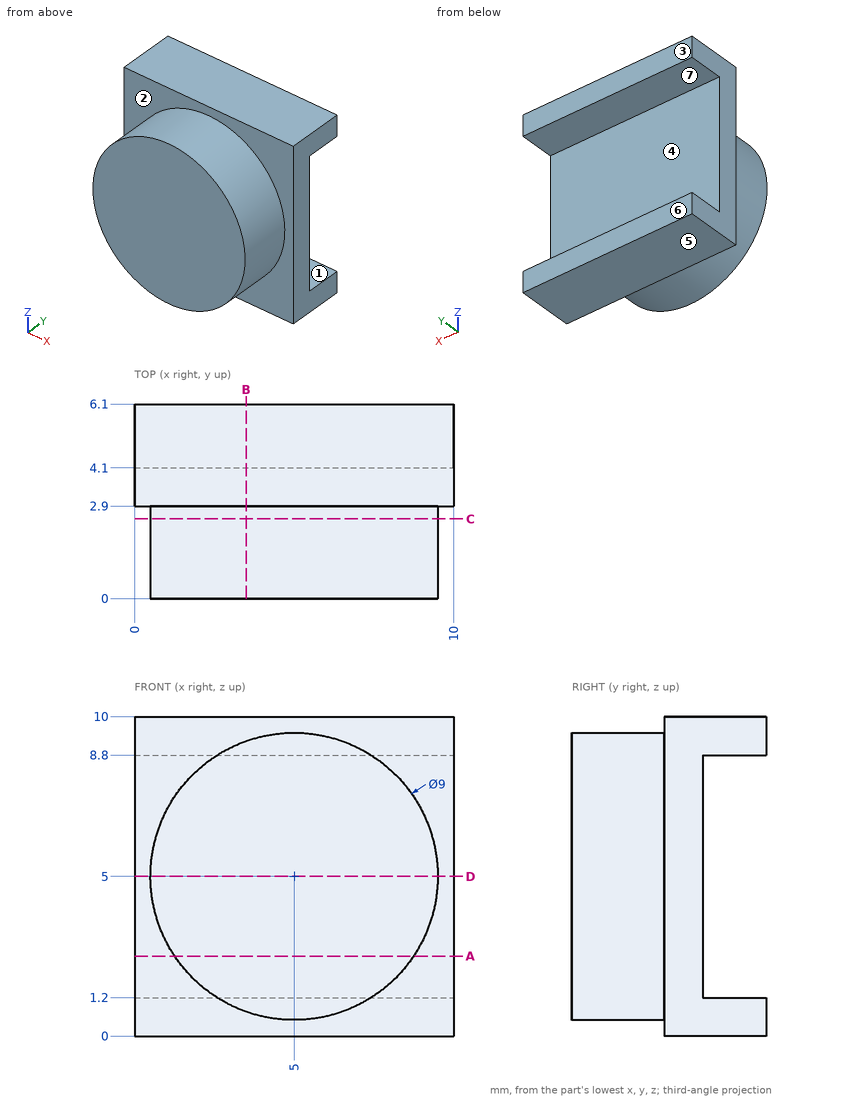
For this review, use the dimensioned drawing (mm, ordinates from the lowest corner) and the shaded views. A direction names the side the tool comes from. Give positions to 0.01 mm unless a question says otherwise; leave off trailing zeros. Loops run counter-clockwise (first coordinate to the right, second up) from the corner with the lowest first, then second, coordinate; pieces in that order, holes last.
Item 1: Take a section at D-D, the plane z = 5. State the section outline as (x, y) points.
Item 2: Tool access review of the marked faces 1, 2 and 3: name each direction out of +Z, -Z, +X, -X, +Y, -Y from which nothing blocks a thin tool from reaching the whole face with its end or side.
Item 3: Take a section at B-B, the plane x = 3.5. State the section outline as (y, z) points, and give its area (3 significant figures).
Item 4: Draft analysis for pull direction Z (two halves, no side actions). For the marked faces 4, 5, 6 and 7, state which applies: +Z half, -Z half, draft (parallel to the pull), parting line (faces both ways), or undercut.
Item 5: Take a section at A-A, the plane z = 2.5. State the section outline as (x, y) points, and give its area (3 significant figures).
Item 6: For line 1 along Z through (x, y) = (6.75, 5.5); line 2 along X through (y, z) = (1, 5); line 3 along Y through (x, z) = (4.5, 2.5), list the stretches that pass through material, from the lowest coordinate up.
Item 7: Take a section at C-C, the plane y = 2.5. State the section outline as (x, z) points.
Item 8: Insertion check: pin 1 (3 mm diameter, centred on x = 6.5, z = 5.5, fed in from +Y). The pin has a flat end and moves straight along its axis. Give the tip position at first contact, or say it passes through.
Calculated:
1. outline: (0, 2.9) - (0.5, 2.9) - (0.5, 0) - (9.5, 0) - (9.5, 2.9) - (10, 2.9) - (10, 4.1) - (0, 4.1) - close
2. face 1: +X, -X, +Y
2. face 2: -Y
2. face 3: +Z, -Z, +X, -X, +Y
3. outline: (0, 0.76) - (2.9, 0.76) - (2.9, 0) - (6.1, 0) - (6.1, 1.2) - (4.1, 1.2) - (4.1, 8.8) - (6.1, 8.8) - (6.1, 10) - (2.9, 10) - (2.9, 9.24) - (0, 9.24) - close
3. area: 41.4 mm2
4. face 4: undercut
4. face 5: -Z half
4. face 6: draft
4. face 7: undercut
5. outline: (0, 2.9) - (1.26, 2.9) - (1.26, 0) - (8.74, 0) - (8.74, 2.9) - (10, 2.9) - (10, 4.1) - (0, 4.1) - close
5. area: 33.7 mm2
6. line 1: z = 0 to 1.2, 8.8 to 10
6. line 2: x = 0.5 to 9.5
6. line 3: y = 0 to 4.1
7. outline: circle Ø9 at (5, 5)
8. pin 1: stops at y = 4.1
